Autodesk Inventor part; units mm, degrees
ref_plane "YZ Plane" through (0, 0, 0) normal (1, 0, 0) x (0, 1, 0)
ref_plane "XZ Plane" through (0, 0, 0) normal (0, 1, 0) x (-1, 0, 0)
ref_plane "XY Plane" through (0, 0, 0) normal (0, 0, 1) x (1, 0, 0)
sketch "Sketch1" plane through (0, 0, 0) normal (0, 1, 0) x (-1, 0, 0)
  line L0 (0, 0) -> (0, 300)
  line L1 (0, 300) -> (190, 300)
  line L2 (190, 300) -> (190, 0)
  line L3 (190, 0) -> (0, 0)
  line L4 (0, 300) -> (95, 300)
  line L5 (0, 300) -> (95, 300) construction
  line L6 (95, 300) -> (95, -51.2612)
  point P0 (95, 0)
  dimension "d0" = 300
  dimension "d1" = 190
  dimension "d2" = 90
  dimension "d3" = 300
  dimension "d4" = 90
  dimension "d23" = 95
  dimension "d24" = 0
  dimension "d25" = 90
extrude "Extrusion1" add sketch "Sketch1" along normal blind 3 contours L6 L1 L2 L3
sketch "Sketch2" plane through (0, 3, 0) normal (0, 1, 0) x (1, 0, 0)
  line L0 (-190, 0) -> (-190, -300)
  line L1 (-190, -300) -> (-190, -210)
  line L2 (-190, -210) -> (-190, -200)
  line L3 (-190, -200) -> (-190, -150)
  line L4 (-190, -210) -> (-190, -220)
  line L5 (-190, -150) -> (-150, -150)
  line L6 (-150, -150) -> (-150, -200)
  line L7 (-150, -200) -> (-190, -200)
  line L8 (-190, -200) -> (-190, -150)
  line L9 (-190, -220) -> (-150, -220)
  line L10 (-150, -220) -> (-150, -270)
  line L11 (-150, -270) -> (-190, -270)
  line L12 (-190, -270) -> (-190, -220)
  line L13 (-190, -220) -> (-180, -220)
  line L14 (-180, -220) -> (-180, -200)
  point P0 (0, 0)
  point P1 (-190, -270)
  dimension "d7" = 90
  dimension "d8" = 10
  dimension "d9" = 50
  dimension "d10" = 10
  dimension "d11" = 40
  dimension "d12" = 50
  dimension "d13" = 40
  dimension "d14" = 50
  dimension "d15" = 10
extrude "Extrusion2" cut sketch "Sketch2" against normal blind 3
mirror "Mirror1" about plane through (-95, 0, 300) normal (1, 0, 0) of "Extrusion2", "Extrusion1"
sketch "Sketch4" plane through (0, 3, 0) normal (0, 1, 0) x (1, 0, 0)
  line L0 (-40, -200) -> (-10, -200)
  line L1 (-10, -200) -> (-10, -210)
  line L2 (-10, -200) -> (0, -200) construction
  line L3 (-10, -210) -> (-25, -210)
  line L4 (-180, -200) -> (-180, -210)
  line L5 (-180, -200) -> (-180, -220)
  line L6 (-180, -200) -> (-170, -200) construction
  line L7 (-180, -210) -> (-165, -210)
  circle A0 centre (-165, -210) radius 2
  circle A1 centre (-25, -210) radius 2
  point P0 (0, 0)
  dimension "d26" = 10
  dimension "d27" = 90
  dimension "d28" = 15
  dimension "d29" = 90
  dimension "d30" = 10
  dimension "d31" = 90
  dimension "d32" = 15
  dimension "d33" = 90
  dimension "d34" = 4
  dimension "d35" = 4
extrude "Extrusion4" cut sketch "Sketch4" against normal blind 10
sketch "Sketch5" plane through (0, 3, 0) normal (0, 1, 0) x (1, 0, 0)
  circle A0 centre (-165, -210) radius 2
  line L0 (-165, -210) -> (-95, -210)
  circle A1 centre (-95, -210) radius 0.05
  point P0 (0, 0)
  dimension "d38" = 70
  dimension "d39" = 0.1
extrude "Extrusion5" cut sketch "Sketch5" against normal blind 10 contours A1
properties part number "onderplaat v2"
Could you check a few things on this model? Use its own coordinates, in mm. Round coordinates to 2 decimals unless told otherwise and drop trailing zeros. Order: outer loops, then holes, each group sorted by start corner. A loop starts at its lowest first (then second) coordinate and runs counter-clockwise, first axis right, second up. Notation, with made-up numbers: M -5,0 L 19,0 A33 ccw 19,39 Z; hole C -1,15 d11. An arc over 180 degrees is marked long. One line per question, with ' | ' between items. Start each with the question number.
(1) Please list where these lines run through material, in increasing order: line 1 along Z through (x, y) = (-28, 1.75); line 2 along Z through (x, y) = (-165, 0.6); line 3 along Z through (x, y) = (-182, 2.8).
(2) Suppose I cut it at B-B on z = 179. List the corners of the cut face in (x, y) for me.
(3) For P1, Ø1.5, axis at y = 1.5, z = 234, coming from the -X side, with a flat end and sliding along its axis, tell me the tip position at first contact or that it passes through.
Geometry results:
1) line 1: 0 to 150, 200 to 220, 270 to 300 | line 2: 0 to 150, 200 to 208, 212 to 220, 270 to 300 | line 3: 0 to 150, 270 to 300
2) outline: M -150,0 L -40,0 L -40,3 L -150,3 Z
3) P1: x = -150
